from build123d import *

# Parameters (mm, degrees)
SKETCH_1_W            = 3
SKETCH_1_H            = 12.5
SKETCH_2_R            = 7.5
EXTRUDE_1_DEPTH       = 40
CUT_EXTRUDE_1_DEPTH   = 47.491934784
HOLE_WIZARD_3_0_3_3_D = 3
SKETCH_9_R            = 1.25
CUT_EXTRUDE_2_DEPTH   = 10


with BuildPart() as part:
    # 草图1 → 旋转1 (revolve)
    with BuildSketch(Plane(origin=(0, 0, 0), x_dir=(-1, 0, 0), z_dir=(0, 0, -1)), mode=Mode.PRIVATE) as revolve_1_sk:
        with Locations((-41.5, 6.25)):
            Rectangle(SKETCH_1_W, SKETCH_1_H)
    revolve(revolve_1_sk.sketch.rotate(Axis((43, 0, 0), (-1, 0, 0)), 270), axis=Axis((43, 0, 0), (-1, 0, 0)))

    # 草图2 → 凸台-拉伸1 (add)
    with BuildSketch(Plane.ZY.offset(-40)):
        Circle(SKETCH_2_R)
    extrude(amount=EXTRUDE_1_DEPTH)

    # 草图3 → 切除-拉伸1 (cut, through all)
    with BuildSketch(Plane.ZY):
        with BuildLine():
            Line((3.082612528, 4), (-3.082612528, 4))
            ThreePointArc((-3.082612528, 4), (0, -5.05), (3.082612528, 4))
        make_face()
    extrude(amount=-CUT_EXTRUDE_1_DEPTH, mode=Mode.SUBTRACT)

    # Ø3.0 (3) 直径孔3 (through all)
    with Locations(Plane.ZY.offset(-40)):
        with Locations((10, 0), (0, -10), (-10, 0), (0, 10)):
            Hole(HOLE_WIZARD_3_0_3_3_D / 2)

    # 草图9 → 切除-拉伸2 (cut)
    with BuildSketch(Plane.XZ.offset(-4)):
        with Locations(Location((18, 0, 0), (0, 0, 270))):
            Circle(SKETCH_9_R)
    extrude(amount=-CUT_EXTRUDE_2_DEPTH, mode=Mode.SUBTRACT)


solid = part.part
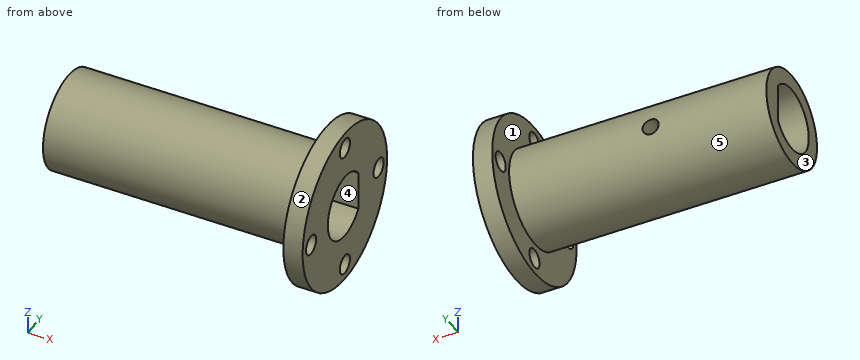
The model under review builds one solid part; all positions refer to its coordinate system, in mm. Face numbers are marked on the shaded views. A direction names the side the tool comes from. Give positions to 0.01 mm unless a question says otherwise; leave off trailing zeros. Write each loop counter-clockwise with the first axis right and the second up, starting at its lowest first coordinate (ties: lowest second). Pieces come first, ordered by that corner, then holes.
1. Add section B-B, the plane y = 0. Write out the cut boundary in (x, z).
2. Add section A-A, the plane z = 0. Write out the cut boundary in (x, y), plus the area to 3 significant figures.
3. Draft analysis for pull direction Y (two halves, no side actions). For the marked faces 3, 4 and 5, state which applies: +Y half, -Y half, draft (parallel to the pull), parting line (faces both ways), or undercut.
4. For P1, Ø1.8, axis at y = 10, z = 0, coming from the +X side; P2, Ø7, axis at x = 28.5, z = 0.5, coming from the -Y side; P3, Ø2, axis at x = 38.5, z = 5.5, coming from the +Y side; P4, Ø3, axis at y = -6.5, z = -8, coming from the -X side, all flat-tipped, find the tip position at first contact; note any pin that passes through.
5. Wall thickness on L1, parallel to Y at x = 41.8, z = 0; L2, parallel to Y at x = 10, z = 0; L3, parallel to Y at x = 41.3, z = 10: over which ranges is each line inside the solid? List them lowest first.
6. Add section C-C, the plane y = 10. Write out the cut boundary in (x, z).
7. Tool access review of the marked faces 1 and 2: name each direction out of +Z, -Z, +X, -X, +Y, -Y from which nothing blocks a thin tool from reaching the whole face with its end or side.
Worked answers:
1. outline: (0, -7.5) - (40, -7.5) - (40, -8.5) - (43, -8.5) - (43, -5.05) - (0, -5.05) - close; (0, 5.05) - (43, 5.05) - (43, 8.5) - (40, 8.5) - (40, 7.5) - (0, 7.5) - close; (40, -12.5) - (43, -12.5) - (43, -11.5) - (40, -11.5) - close; (40, 11.5) - (43, 11.5) - (43, 12.5) - (40, 12.5) - close
2. outline: (0, -7.5) - (40, -7.5) - (40, -8.5) - (43, -8.5) - (43, -5.05) - (0, -5.05) - close; (0, 4) - (16.75, 4) - (16.75, 7.5) - (0, 7.5) - close; (19.25, 4) - (43, 4) - (43, 8.5) - (40, 8.5) - (40, 7.5) - (19.25, 7.5) - close; (40, -12.5) - (43, -12.5) - (43, -11.5) - (40, -11.5) - close; (40, 11.5) - (43, 11.5) - (43, 12.5) - (40, 12.5) - close
2. area: 259 mm2
3. face 3: draft
3. face 4: undercut
3. face 5: parting line
4. P1: passes through
4. P2: stops at y = -7.5
4. P3: stops at y = 6
4. P4: stops at x = 40
5. L1: y = -12.5 to -11.5, -8.5 to -5.05, 4 to 8.5, 11.5 to 12.5
5. L2: y = -7.5 to -5.05, 4 to 7.5
5. L3: y = -7.5 to -1.5, 1.5 to 7.5
6. outline: (40, -7.5) - (43, -7.5) - (43, -1.5) - (40, -1.5) - close; (40, 1.5) - (43, 1.5) - (43, 7.5) - (40, 7.5) - close
7. face 1: -X
7. face 2: +X, -X
